```python
from build123d import *

# Parameters (mm, degrees)
SKETCH1_W      = 214.001476942
SKETCH1_H      = 336.63984765
EXTRUDE1_DEPTH = 12.7
SKETCH2_R      = 7.14375
EXTRUDE2_DEPTH = 50.744786622


with BuildPart() as part:
    # Sketch1 → Extrude1 (new body)
    with BuildSketch(Plane(origin=(0, 0, 0), x_dir=(1, 0, 0), z_dir=(0, 1, 0))):
        Rectangle(SKETCH1_W, SKETCH1_H)
    extrude(amount=-EXTRUDE1_DEPTH)

    # Sketch2 → Extrude2 (add)
    with BuildSketch(Plane(origin=(0, 0, 0), x_dir=(-1, 0, 0), z_dir=(0, 1, 0))):
        with BuildLine():
            Line((-35.873271056, 88.9), (-35.873271056, -88.9))
            ThreePointArc((-35.873271056, -88.9), (-33.083463147, -95.635192091), (-26.348271056, -98.425))
            Line((-26.348271056, -98.425), (21.276728944, -98.425))
            ThreePointArc((21.276728944, -98.425), (28.011921035, -95.635192091), (30.801728944, -88.9))
            Line((30.801728944, -88.9), (30.801728944, 88.9))
            ThreePointArc((30.801728944, 88.9), (28.011921035, 95.635192091), (21.276728944, 98.425))
            Line((21.276728944, 98.425), (-26.348271056, 98.425))
            ThreePointArc((-26.348271056, 98.425), (-33.083463147, 95.635192091), (-35.873271056, 88.9))
        make_face()
        with Locations(Location((-2.535771056, 61.9125, 0), (0, 0, 90))):
            Circle(SKETCH2_R, mode=Mode.SUBTRACT)
        with Locations(Location((-2.535771056, -61.9125, 0), (0, 0, 90))):
            Circle(SKETCH2_R, mode=Mode.SUBTRACT)
    extrude(amount=EXTRUDE2_DEPTH)


solid = part.part
```
For this review, take the finished solid that the model builds, in its own axes (mm). A direction names the side the tool comes from. Round coordinates to 2 decimals unless told otherwise and drop trailing zeros. Order: outer loops, then holes, each group sorted by start corner. A loop starts at its lowest first (then second) coordinate and runs counter-clockwise, first axis right, second up.
Q1. We need section B-B, the plane x = 18.5. Give the boundary of the cut face in (y, z) (3 decimals).
Findings below:
outline: (-12.7, -168.32) - (0, -168.32) - (0, -98.425) - (50.745, -98.425) - (50.745, 98.425) - (0, 98.425) - (0, 168.32) - (-12.7, 168.32) - close
Q2. We need section D-D, the plane x = -48. Give the boundary of the cut face in (y, z).
Findings below:
outline: (-12.7, -168.32) - (0, -168.32) - (0, 168.32) - (-12.7, 168.32) - close
Q3. Mouldability with a two-part tool opening along X and no side actions: class faces 1 (the flat face through (107.001, -6, 2)), 2 (the cylindrical face through (2.85, 25.02, -69.05)), 3 (the flat face through (2, 0, 62)), 4 (the flat face through (2, 25, 98.425)) as pulls with the +X half, pulls with the -X half, needs draft (parallel to the pull), parting line crosses it, or undercut.
Findings below:
face 1: pulls with the +X half
face 2: undercut
face 3: undercut
face 4: needs draft
Q4. We need section C-C, the plane y = 27.5. State how many separate pieces and enclosed holes the cut face has, plus the area to 3 significant figures.
Findings below:
separate pieces: 1
enclosed holes: 2
area: 12,700 mm2
Q5. Wall thickness on line 1 (Y direction, x = 24.5, z = -153.5); line 2 (X direction, y = 21.5, z = -78.5); line 3 (X direction, y = 24.5, z = 94.5): over which ranges is each line inside the solid? List them lowest first.
Findings below:
line 1: y = -12.7 to 0
line 2: x = -30.8 to 35.87
line 3: x = -28.98 to 34.05
Q6. We need section A-A, the plane z = -2. Give the boundary of the cut face in (x, y), plus the area to 3 significant figures.
Findings below:
outline: (-107, -12.7) - (107, -12.7) - (107, 0) - (35.87, 0) - (35.87, 50.74) - (-30.8, 50.74) - (-30.8, 0) - (-107, 0) - close
area: 6,100 mm2
Q7. Insertion check: P1, Ø15, axis at y = 23, z = 31.5, coming from the +X side; P2, Ø7, axis at x = 1.5, z = -64.5, coming from the +Y side; P3, Ø14.5, axis at x = -5, y = 20.5, coming from the +Z side (3 decimals). Each pin has a flat end and moves straight along its axis. Give the tip position at first contact, or say it passes through.
Findings below:
P1: stops at x = 35.87
P2: stops at y = 0
P3: stops at z = 98.425
Q8. Machinability: for faces 5 (the cylindrical face through (-27.937, 25.017, -95.709)), 6 (the cylindrical face through (33.16, 25.02, -95.56)), 7 (the flat face through (2, 0, -62)), 8 (the cylindrical face through (-28.086, 25.017, 95.561)), which of the approach directions +Z, -Z, +X, -X, +Y, -Y give a long, thin tool a straight path to every point of the face, cutting with its end or side? Answer none if there is none.
Findings below:
face 5: -Z, -X, +Y
face 6: -Z, +X, +Y
face 7: +Y
face 8: +Z, -X, +Y
